```python
from build123d import *

# Parameters (mm, degrees)
BOSS_EXTRU_1_DEPTH      = 4
D_GAGEMENT_M2_51_D      = 2.9
D_GAGEMENT_M2_51_DEPTH  = 5
D_GAGEMENT_M2_51_TIP    = 0.871247898
D_GAGEMENT_M31_D        = 3.4
D_GAGEMENT_M31_DEPTH    = 6
D_GAGEMENT_M31_TIP      = 1.021463052
D_GAGEMENT_M32_D        = 3.4
D_GAGEMENT_M32_DEPTH    = 5
D_GAGEMENT_M32_TIP      = 1.021463052
ENL_V_MAT_EXTRU_1_DEPTH = 1
ESQUISSE10_3_R          = 1.7
ENL_V_MAT_EXTRU_2_DEPTH = 1
D_GAGEMENT_M33_D        = 3.4
D_GAGEMENT_M33_DEPTH    = 6
D_GAGEMENT_M33_TIP      = 1.021463052
D_GAGEMENT_M34_D        = 3.4
D_GAGEMENT_M34_DEPTH    = 5
D_GAGEMENT_M34_TIP      = 1.021463052
D_GAGEMENT_M35_D        = 3.4
D_GAGEMENT_M35_DEPTH    = 5
D_GAGEMENT_M35_TIP      = 1.021463052


with BuildPart() as part:
    # Esquisse1 → Boss.-Extru.1 (new body)
    with BuildSketch(Plane.XY):
        with BuildLine():
            Line((-87.472008168, 59.584338106), (-117.472008168, 59.584338106))
            Line((-117.472008168, 59.584338106), (-159.472008168, 42.084338106))
            Line((-159.472008168, 42.084338106), (-165.722008168, 27.084338106))
            Line((-165.722008168, 27.084338106), (-165.722008168, -68.315661894))
            Line((-165.722008168, -68.315661894), (-159.472008168, -83.315661894))
            Line((-159.472008168, -83.315661894), (-117.472008168, -100.815661894))
            Line((-117.472008168, -100.815661894), (-87.472008168, -100.815661894))
            ThreePointArc((-87.472008168, -100.815661894), (-80.091099054, -82.996571008), (-62.272008168, -75.615661894))
            Line((-62.272008168, -75.615661894), (47.327991832, -75.615661894))
            ThreePointArc((47.327991832, -75.615661894), (65.147082718, -82.996571008), (72.527991832, -100.815661894))
            Line((72.527991832, -100.815661894), (93.527991832, -95.815661894))
            Line((93.527991832, -95.815661894), (131.527991832, -72.815661894))
            Line((131.527991832, -72.815661894), (161.027991832, -42.815661894))
            Line((161.027991832, -42.815661894), (161.027991832, 1.684338106))
            Line((161.027991832, 1.684338106), (131.527991832, 31.184338106))
            Line((131.527991832, 31.184338106), (93.527991832, 54.184338106))
            Line((93.527991832, 54.184338106), (72.527991832, 59.584338106))
            ThreePointArc((72.527991832, 59.584338106), (65.147082718, 41.76524722), (47.327991832, 34.384338106))
            Line((47.327991832, 34.384338106), (-62.272008168, 34.384338106))
            ThreePointArc((-62.272008168, 34.384338106), (-80.091099054, 41.76524722), (-87.472008168, 59.584338106))
        make_face()
    extrude(amount=BOSS_EXTRU_1_DEPTH)

    # D_gagement M2.51
    with Locations(Plane(origin=(0, 0, 0), x_dir=(-1, 0, 0), z_dir=(0, 0, -1))):
        with Locations((-21.027991832, -8.66564946), (-39.027991832, -8.66564946), (35.972008168, -32.565674331), (53.972008168, -32.565674331)):
            Hole(D_GAGEMENT_M2_51_D / 2, depth=D_GAGEMENT_M2_51_DEPTH)
            with Locations((0, 0, -(D_GAGEMENT_M2_51_DEPTH + D_GAGEMENT_M2_51_TIP / 2))):  # 118° drill point
                Cone(0, D_GAGEMENT_M2_51_D / 2, D_GAGEMENT_M2_51_TIP, mode=Mode.SUBTRACT)

    # D_gagement M31
    with Locations(Plane(origin=(0, 0, 0), x_dir=(-1, 0, 0), z_dir=(0, 0, -1))):
        with Locations((17.896581687, 16.134338106), (-2.752565352, 16.134338106), (53.972008168, -32.565674331), (35.972008168, -32.565674331), (18.196581687, -57.365661894), (-2.452565352, -57.365661894), (-39.027991832, -8.66564946), (-21.027991832, -8.66564946)):
            Hole(D_GAGEMENT_M31_D / 2, depth=D_GAGEMENT_M31_DEPTH)
            with Locations((0, 0, -(D_GAGEMENT_M31_DEPTH + D_GAGEMENT_M31_TIP / 2))):  # 118° drill point
                Cone(0, D_GAGEMENT_M31_D / 2, D_GAGEMENT_M31_TIP, mode=Mode.SUBTRACT)

    # D_gagement M32
    with Locations(Plane(origin=(0, 0, 0), x_dir=(-1, 0, 0), z_dir=(0, 0, -1))):
        with Locations((69.972008168, -62.728910548), (69.972008168, 21.49758676), (-65.027991832, -62.728910548), (-65.027991832, 21.49758676)):
            Hole(D_GAGEMENT_M32_D / 2, depth=D_GAGEMENT_M32_DEPTH)
            with Locations((0, 0, -(D_GAGEMENT_M32_DEPTH + D_GAGEMENT_M32_TIP / 2))):  # 118° drill point
                Cone(0, D_GAGEMENT_M32_D / 2, D_GAGEMENT_M32_TIP, mode=Mode.SUBTRACT)

    # Esquisse10 → Enl_v. mat.-Extru.1 (cut)
    with BuildSketch(Plane.XY.offset(4)):
        Polygon((43.027991832, -75.615661894), (43.027991832, -70.615661894), (12.42027445, -70.615661894), (12.42027445, -50.615661894), (-27.372008168, -50.615661894), (-27.372008168, -70.615661894), (-36.072008168, -70.615661894), (-39.872008168, -70.615661894), (-39.872008168, -38.615661894), (-50.072008168, -38.615661894), (-50.072008168, -70.615661894), (-57.972008168, -70.615661894), (-57.972008168, -75.615661894), align=None)
    extrude(amount=-ENL_V_MAT_EXTRU_1_DEPTH, mode=Mode.SUBTRACT)

    # Esquisse10_3 → Enl_v. mat.-Extru.2 (cut)
    with BuildSketch(Plane.XY.offset(4)):
        Polygon((43.027991832, 29.384338106), (43.027991832, 34.384338106), (-57.972008168, 34.384338106), (-57.972008168, 29.384338106), (-27.572008168, 29.384338106), (-27.572008168, 9.384338106), (12.427991832, 9.384338106), (12.427991832, 29.384338106), (24.927991832, 29.384338106), (24.927991832, -2.615661894), (35.127991832, -2.615661894), (35.127991832, 29.384338106), align=None)
        with Locations(Location((-17.896581687, 16.134338106, 0), (0, 0, 180.000000005))):
            Circle(ESQUISSE10_3_R, mode=Mode.SUBTRACT)
        with Locations(Location((2.752565352, 16.134338106, 0), (0, 0, 180.000000005))):
            Circle(ESQUISSE10_3_R, mode=Mode.SUBTRACT)
    extrude(amount=-ENL_V_MAT_EXTRU_2_DEPTH, mode=Mode.SUBTRACT)

    # D_gagement M33
    with Locations(Plane(origin=(0, 0, 0), x_dir=(-1, 0, 0), z_dir=(0, 0, -1))):
        with Locations((104.471408589, -30.715661894), (129.871408589, 24.484338106)):
            Hole(D_GAGEMENT_M33_D / 2, depth=D_GAGEMENT_M33_DEPTH)
            with Locations((0, 0, -(D_GAGEMENT_M33_DEPTH + D_GAGEMENT_M33_TIP / 2))):  # 118° drill point
                Cone(0, D_GAGEMENT_M33_D / 2, D_GAGEMENT_M33_TIP, mode=Mode.SUBTRACT)

    # D_gagement M34
    with Locations(Plane(origin=(0, 0, 0), x_dir=(-1, 0, 0), z_dir=(0, 0, -1))):
        with Locations((-100.527991832, -41.815661894), (-115.527991832, -41.815661894), (-100.527991832, -12.115661894), (-115.527991832, -12.115661894)):
            Hole(D_GAGEMENT_M34_D / 2, depth=D_GAGEMENT_M34_DEPTH)
            with Locations((0, 0, -(D_GAGEMENT_M34_DEPTH + D_GAGEMENT_M34_TIP / 2))):  # 118° drill point
                Cone(0, D_GAGEMENT_M34_D / 2, D_GAGEMENT_M34_TIP, mode=Mode.SUBTRACT)

    # D_gagement M35
    with Locations(Plane(origin=(0, 0, 0), x_dir=(-1, 0, 0), z_dir=(0, 0, -1))):
        with Locations((150.085256822, -69.115661894), (83.358759514, -69.115661894)):
            Hole(D_GAGEMENT_M35_D / 2, depth=D_GAGEMENT_M35_DEPTH)
            with Locations((0, 0, -(D_GAGEMENT_M35_DEPTH + D_GAGEMENT_M35_TIP / 2))):  # 118° drill point
                Cone(0, D_GAGEMENT_M35_D / 2, D_GAGEMENT_M35_TIP, mode=Mode.SUBTRACT)


solid = part.part
```
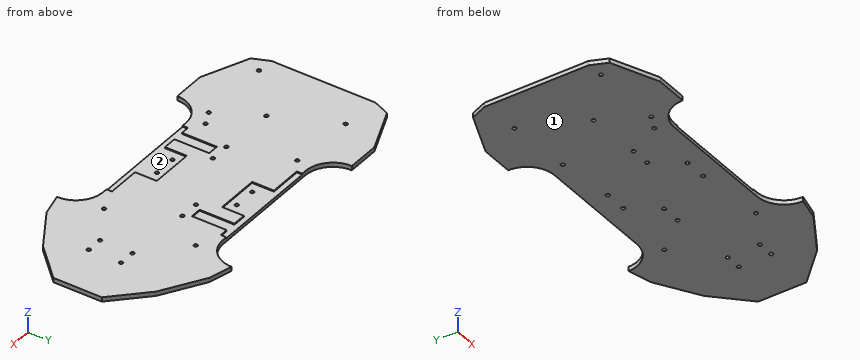
The model under review builds one solid part; all positions refer to its coordinate system, in mm. Face numbers are marked on the shaded views. Give positions to 0.01 mm unless a question says otherwise; leave off trailing zeros. Write each loop counter-clockwise with the first axis right and the second up, starting at its lowest first coordinate (ties: lowest second). Pieces come first, ordered by that corner, then holes. Notation, with made-up numbers: (56, -13) -> (110, -13) arc R19 ccw to (110, 9) -> close; hole circle Ø2 at (82.25, 62). An arc over 180 degrees is marked (long way). Answer in a Markdown table with one row per item.
1) Add section C-C on y = -79. State the section outline as (x, z) points.
Worked answers:
| item | result |
|---|---|
| outline | (-161.27, 0) -> (-74.89, 0) -> (-74.89, 4) -> (-161.27, 4) -> close; (59.94, 0) -> (121.31, 0) -> (121.31, 4) -> (59.94, 4) -> close |
2) Add section A-A on y = 50.5. State the section outline as (x, z) points.
Worked answers:
| item | result |
|---|---|
| outline | (-139.27, 0) -> (-85.78, 0) -> (-85.78, 4) -> (-139.27, 4) -> close; (70.83, 0) -> (99.62, 0) -> (99.62, 4) -> (70.83, 4) -> close |
3) For L1, parallel to Y at x = 114, z = 1.6; L2, parallel to X at y = -42.5, z = 2.9; L3, parallel to X at y = -11.5, z = 3.4, list the stretches that pass through material, from the lowest coordinate up. Write a range as [from, to].
Worked answers:
| item | result |
|---|---|
| L1 | [-83.42, -42.56], [-41.07, -12.86], [-11.37, 41.79] |
| L2 | [-165.72, 98.97], [102.08, 113.97], [117.08, 161.03] |
| L3 | [-165.72, 98.94], [102.11, 113.94], [117.11, 161.03] |
4) Add section D-D on z = 1.3. Count the separate pieces of the cut face and the enclosed holes in it, plus the area to 3 significant figures.
Worked answers:
| item | result |
|---|---|
| separate pieces | 1 |
| enclosed holes | 20 |
| area | 39,700 mm² |
5) Add section B-B on x = -120.5. State the section outline as (y, z) points.
Worked answers:
| item | result |
|---|---|
| outline | (-99.55, 0) -> (58.32, 0) -> (58.32, 4) -> (-99.55, 4) -> close |
6) Mouldability with a two-part tool opening along X and no side actions: class the marked faces 1 and 2 as +X half, -X half, draft (parallel to the pull), parting line (faces both ways), or undercut.
Worked answers:
| item | result |
|---|---|
| face 1 | draft |
| face 2 | undercut |
7) Clearance check with flat-ended pins moving along their axes: P1, Ø1.5, axis at x = -21.5, y = 22, coming from the +Z side; P2, Ø1.5, axis at x = 100, z = 3, coming from the -Y side; P3, Ø2.5, axis at x = -69.97, y = -62.73, coming from the +Z side; P4, Ø0.5, axis at y = 31.5, z = 3.5, coming from the -X side. State where each tip first meets the part, or that it passes through.
Worked answers:
| item | result |
|---|---|
| P1 | z = 3 |
| P2 | y = -92.35 |
| P3 | through |
| P4 | x = -163.99 |
